```python
from build123d import *

# Parameters (mm, degrees)
F1_DEPTH = 25.4
F3_DEPTH = 25.4
F4_T     = -2.54


with BuildPart() as f1:
    # F0 (on Top) → F1 (new body)
    with BuildSketch(Plane.XY):
        with BuildLine():
            Line((19.2348733544, 7.6057617553), (-35.5748815684, 7.6057617553))
            ThreePointArc((-35.5748815684, 7.6057617553), (-75.5952649714, -15.9430811399), (-121.9473853707, -18.71075596))
            Line((-121.9473853707, -18.71075596), (-121.9473853707, -56.1465583742))
            Line((-121.9473853707, -56.1465583742), (19.2348733544, -56.1465583742))
            Line((19.2348733544, -56.1465583742), (19.2348733544, 7.6057617553))
        make_face()
        with BuildLine():
            Line((-35.5748815684, 7.6057617553), (-121.9473853707, 7.6057617553))
            Line((-121.9473853707, 7.6057617553), (-121.9473853707, -18.71075596))
            ThreePointArc((-121.9473853707, -18.71075596), (-75.5952649714, -15.9430811399), (-35.5748815684, 7.6057617553))
        make_face()
        with BuildLine():
            Line((-121.9473853707, -18.71075596), (-121.9473853707, 7.6057617553))
            Line((-121.9473853707, 7.6057617553), (-35.5748815684, 7.6057617553))
            ThreePointArc((-35.5748815684, 7.6057617553), (-13.1607449358, 40.2200486566), (-5.2712796474, 78.9994448423))
            ThreePointArc((-5.2712796474, 78.9994448423), (-168.2469260973, 155.0924750547), (-121.9473853707, -18.71075596))
        make_face()
    extrude(amount=F1_DEPTH)

    # F2 (on face) → F3 (join)
    with BuildSketch(Plane.XY.offset(25.4)):
        with BuildLine():
            ThreePointArc((-149.3627248428, -9.5459612091), (-95.718013043, 19.6715775936), (-74.3504000093, 76.8978372216))
            ThreePointArc((-74.3504000093, 76.8978372216), (-97.8658435535, 136.509233554), (-155.7459184192, 164.0118078208))
            ThreePointArc((-155.7459184192, 164.0118078208), (-203.7075635009, 75.3515840449), (-149.3627248428, -9.5459612091))
        make_face()
    extrude(amount=-F3_DEPTH)

    # F4
    f4_openings = [f1.faces().sort_by_distance(p)[0] for p in [
        (-92.78675, 58.561614, 0),
    ]]
    offset(amount=F4_T, openings=f4_openings, kind=Kind.INTERSECTION)


solid = f1.part
```
The model under review builds one solid part; all positions refer to its coordinate system, in mm. A direction names the side the tool comes from. Coordinates: 2 decimals unless noted, no trailing zeros. Write each loop counter-clockwise with the first axis right and the second up, starting at its lowest first coordinate (ties: lowest second). Pieces come first, ordered by that corner, then holes. Notation, with made-up numbers: (-27, 86) -> (29, 86) arc R37 cw to (29, 122) -> close; hole circle Ø4 at (-31, 40.25). An arc over 180 degrees is marked (long way). One line per item, written item: value. Start each with the question number.
Q1. The part is to be moulded in two halves that separate along Y. For faces 1 (the face through (-94, 63, 22.86)), 2 (the face through (-52, -56.147, 13)), 3 (the face through (-121.947, -37, 13)), say which applies: +Y half, -Y half, draft (parallel to the pull), parting line (faces both ways), or undercut.
Q2. Add section C-C, the plane x = -94. Give the boundary of the cut face in (y, z).
Q3. Add section A-A, the plane z = 5.75. Give the boundary of the cut face in (x, y), then the cut area to 3 significant figures.
Q4. Add section B-B, the plane y = 72.5. Give the boundary of the cut face in (x, z).
Q5. For faces 4 (the face through (-8, 7.606, 13)), 5 (the face through (-119.407, -35, 11)), 6 (the face through (-192, 122, 0)), list the 3-axis set-ups (+Z, -Z, +X, -X, +Y, -Y) from which the entire face can be reached by the end or side of a thin tool; tool diameter is ignored.
Q6. To check wall thickness, follow probe 1 along X at (y, z) = (-19, 11.25); probe 2 along Y at (x, z) = (5, 11.75); probe 3 along Y at (x, z) = (-31, 19). State the ranges of each line that lie inside material, in increasing order.
Q7. Clearance check with flat-ended pins moving along their axes: P1, Ø1.5, axis at y = -1.5, z = 14.5, coming from the -X side; P2, Ø8, axis at x = -76, z = 5, coming from the +Y side; P3, Ø11.5, axis at x = -57.5, z = 7.5, coming from the +Y side. State where each tip first meets the part, or that it passes through.
Response:
1. face 1: undercut
1. face 2: -Y half
1. face 3: draft
2. outline: (-56.15, 0) -> (-53.61, 0) -> (-53.61, 22.86) -> (175.14, 22.86) -> (175.14, 0) -> (177.69, 0) -> (177.69, 25.4) -> (-56.15, 25.4) -> close
3. outline: (-121.95, -56.15) -> (19.23, -56.15) -> (19.23, 7.61) -> (-35.57, 7.61) arc R99.25 ccw (long way) to (-121.95, -18.71) -> close; hole (-119.41, -53.61) -> (16.69, -53.61) -> (16.69, 5.07) -> (-42.18, 5.07) arc R96.71 ccw (long way) to (-119.41, -16.56) -> close
3. area: 2,090 mm²
4. outline: (-203.56, 0) -> (-201.02, 0) -> (-201.02, 22.86) -> (-8.03, 22.86) -> (-8.03, 0) -> (-5.48, 0) -> (-5.48, 25.4) -> (-203.56, 25.4) -> close
5. face 4: +Z, -Z, +X
5. face 5: -Z
5. face 6: -Z, +X, -X, +Y, -Y
6. probe 1: -121.95 to -119.41, 16.69 to 19.23
6. probe 2: -56.15 to -53.61, 5.07 to 7.61
6. probe 3: -56.15 to -53.61, 5.07 to 7.61, 12.33 to 16.17, 141.83 to 145.67
7. P1: x = -163.61
7. P2: y = 175.17
7. P3: y = 169.26
